Read the model definition and answer for the solid it produces. Units are mm, in the model's axes. A direction names the side the tool comes from. Coordinates: 2 decimals unless noted, no trailing zeros. Write each loop counter-clockwise with the first axis right and the second up, starting at its lowest first coordinate (ties: lowest second). Pieces come first, ordered by that corner, then holes. Notation, with made-up numbers: (62, 33.5) -> (113, 33.5) arc R22 ccw to (113, 64.5) -> close; hole circle Ø11 at (75.25, -11.75). An arc over 180 degrees is marked (long way). Return JSON: item names as keys, results as strings.
from build123d import *

# Parameters (mm, degrees)
SKETCH_1_W          = 28
SKETCH_1_H          = 31.376198505
SKETCH_1_R          = 1.25
EXTRUDE_1_DEPTH     = 4
SKETCH_4_R          = 2
EXTRUDE_3_DEPTH     = 3
SKETCH_6_R          = 2
EXTRUDE_4_DEPTH     = 24.38
SKETCH_7_W          = 28
SKETCH_7_H          = 2
CUT_EXTRUDE_1_DEPTH = 72


with BuildPart() as part:
    # 草图1 → 凸台-拉伸1 (new body)
    with BuildSketch(Plane.XY):
        with Locations((0, -1.688099253)):
            Rectangle(SKETCH_1_W, SKETCH_1_H)
        with Locations((-12, -12)):
            Circle(SKETCH_1_R, mode=Mode.SUBTRACT)
        with Locations((-12, 12)):
            Circle(SKETCH_1_R, mode=Mode.SUBTRACT)
        with Locations((12, 12)):
            Circle(SKETCH_1_R, mode=Mode.SUBTRACT)
        with Locations((12, -12)):
            Circle(SKETCH_1_R, mode=Mode.SUBTRACT)
    extrude(amount=EXTRUDE_1_DEPTH)

    # 草图4 → 凸台-拉伸3 (add)
    with BuildSketch(Plane(origin=(0, -17.376198505, 0), x_dir=(1, 0, 0), z_dir=(0, 1, 0))):
        with BuildLine():
            Line((-10.75, -4), (-16.6423045, -25.198978267))
            ThreePointArc((-16.6423045, -25.198978267), (-17.942800458, -27.122401454), (-20.139772651, -27.873507091))
            Line((-20.139772651, -27.873507091), (-24.991319672, -27.873507091))
            ThreePointArc((-24.991319672, -27.873507091), (-26.405533234, -27.287720654), (-26.991319672, -25.873507091))
            Line((-26.991319672, -25.873507091), (-26.991319672, -23.098090883))
            ThreePointArc((-26.991319672, -23.098090883), (-26.405533234, -21.68387732), (-24.991319672, -21.098090883))
            Line((-24.991319672, -21.098090883), (-20.272369191, -21.098090883))
            ThreePointArc((-20.272369191, -21.098090883), (-19.062245191, -20.690447597), (-18.345420115, -19.633690786))
            Line((-18.345420115, -19.633690786), (-14, -4))
            Line((-14, -4), (-10.75, -4))
        make_face()
        with Locations((-21, -24)):
            Circle(SKETCH_4_R, mode=Mode.SUBTRACT)
    extrude_3 = extrude(amount=EXTRUDE_3_DEPTH)

    # 草图6 → 凸台-拉伸4 (add)
    with BuildSketch(Plane(origin=(0, -14.376198505, 0), x_dir=(1, 0, 0), z_dir=(0, 1, 0))):
        with BuildLine():
            ThreePointArc((-20.272369191, -21.098090883), (-17.534000745, -22.331206649), (-16.6423045, -25.198978267))
            ThreePointArc((-16.6423045, -25.198978267), (-17.942800458, -27.122401454), (-20.139772651, -27.873507091))
            Line((-20.139772651, -27.873507091), (-24.991319672, -27.873507091))
            ThreePointArc((-24.991319672, -27.873507091), (-26.405533234, -27.287720654), (-26.991319672, -25.873507091))
            Line((-26.991319672, -25.873507091), (-26.991319672, -23.098090883))
            ThreePointArc((-26.991319672, -23.098090883), (-26.405533234, -21.68387732), (-24.991319672, -21.098090883))
            Line((-24.991319672, -21.098090883), (-20.272369191, -21.098090883))
        make_face()
        with Locations((-21, -24)):
            Circle(SKETCH_6_R, mode=Mode.SUBTRACT)
    extrude_4 = extrude(amount=EXTRUDE_4_DEPTH)

    # 镜向1: 凸台-拉伸3, 凸台-拉伸4 across plane
    add(extrude_3.mirror(Plane(origin=(0, 0, 0), x_dir=(0, 0, 1), z_dir=(1, 0, 0))))
    add(extrude_4.mirror(Plane(origin=(0, 0, 0), x_dir=(0, 0, 1), z_dir=(1, 0, 0))))

    # 草图7 → 切除-拉伸1 (cut)
    with BuildSketch(Plane(origin=(0, 14, 0), x_dir=(1, 0, 0), z_dir=(0, 1, 0))):
        with Locations((0, -1)):
            Rectangle(SKETCH_7_W, SKETCH_7_H)
    extrude(amount=-CUT_EXTRUDE_1_DEPTH, mode=Mode.SUBTRACT)


solid = part.part
1. Flat-ended cylindrical pins translate along their axes: pin 1 Ø3 at (x, y) = (12, -12) entering from +Z; pin 2 Ø12 at (y, z) = (10, 9.5) entering from -X; pin 3 Ø2 at (y, z) = (-8.5, 3.5) entering from +X; pin 4 Ø2 at (x, y) = (-12, 12) entering from +Z. Find the tip coordinate at first contact, or state that the pin passes through.
Taken from the geometry:
{"pin 1": "stops at z = 4", "pin 2": "stops at x = -14", "pin 3": "stops at x = 14", "pin 4": "passes through"}
2. For a pull along X with two mould halves and no side action, classify faces 3 (the face through (26.42, -3.88, 21.7)), 4 (the face through (11.84, 13.24, 2.99)), 5 (the face through (0, -1, 2)), 6 (the face through (-22.474, -3.878, 22.648)) as +X half, -X half, draft (parallel to the pull), parting line (faces both ways), or undercut.
Taken from the geometry:
{"face 3": "+X half", "face 4": "undercut", "face 5": "draft", "face 6": "undercut"}
3. A tool of negligible diameter and unlimited length cuts with its end or side. For faces 1 (the face through (-17.917, -3.878, 27.102)), 2 (the face through (-23, 10.004, 25)), from which of +Z, -Z, +X, -X, +Y, -Y can it reach the whole face along a straight path? Write none if from no direction.
Taken from the geometry:
{"face 1": "+Z, +Y, -Y", "face 2": "+Z, -Z, +X, -X, +Y"}
4. Consider L1, parallel to X at y = -12, z = 2.45; L2, parallel to Y at x = -12, z = 3.1; L3, parallel to Z at x = 21, y = -11. Determine where each line is inside the solid, lowest interval first.
Taken from the geometry:
{"L1": "x = -14 to -13.25, -10.75 to 10.75, 13.25 to 14", "L2": "y = -17.38 to -13.25, -10.75 to 10.75, 13.25 to 14", "L3": "z = 21.1 to 22, 26 to 27.87"}
5. The part is cut by section C-C (y = -12). Determine the outline of the cut face in (x, z), then the cut area to 3 significant figures.
Taken from the geometry:
{"outline": "(-26.99, 23.1) arc R2 ccw to (-24.99, 21.1) -> (-20.27, 21.1) arc R3.66 ccw to (-16.64, 25.2) arc R3.65 ccw to (-20.14, 27.87) -> (-24.99, 27.87) arc R2 ccw to (-26.99, 25.87) -> close; (-14, 2) -> (-13.25, 2) -> (-13.25, 4) -> (-14, 4) -> close; (-10.75, 2) -> (10.75, 2) -> (10.75, 4) -> (-10.75, 4) -> close; (13.25, 2) -> (14, 2) -> (14, 4) -> (13.25, 4) -> close; (16.64, 25.2) arc R3.66 ccw to (20.27, 21.1) -> (24.99, 21.1) arc R2 ccw to (26.99, 23.1) -> (26.99, 25.87) arc R2 ccw to (24.99, 27.87) -> (20.14, 27.87) arc R3.65 ccw to start; hole circle Ø4 at (-21, 24); hole circle Ø4 at (21, 24)", "area": "147 mm2"}
6. The part is cut by section A-A (y = 9). Determine the outline of the cut face in (x, z), then the cut area to 3 significant figures.
Taken from the geometry:
{"outline": "(-26.99, 23.1) arc R2 ccw to (-24.99, 21.1) -> (-20.27, 21.1) arc R3.66 ccw to (-16.64, 25.2) arc R3.65 ccw to (-20.14, 27.87) -> (-24.99, 27.87) arc R2 ccw to (-26.99, 25.87) -> close; (-14, 2) -> (14, 2) -> (14, 4) -> (-14, 4) -> close; (16.64, 25.2) arc R3.66 ccw to (20.27, 21.1) -> (24.99, 21.1) arc R2 ccw to (26.99, 23.1) -> (26.99, 25.87) arc R2 ccw to (24.99, 27.87) -> (20.14, 27.87) arc R3.65 ccw to start; hole circle Ø4 at (-21, 24); hole circle Ø4 at (21, 24)", "area": "157 mm2"}
7. The part is cut by section B-B (x = 21). Determine the outline of the cut face in (y, z), then the cut area to 3 significant figures.
Taken from the geometry:
{"outline": "(-17.38, 21.1) -> (10, 21.1) -> (10, 22) -> (-17.38, 22) -> close; (-17.38, 26) -> (10, 26) -> (10, 27.87) -> (-17.38, 27.87) -> close", "area": "76.0 mm2"}
8. The part is cut by section D-D (z = 18.25). Determine the outline of the cut face in (x, y).
Taken from the geometry:
{"outline": "(-17.96, -17.38) -> (-14.71, -17.38) -> (-14.71, -14.38) -> (-17.96, -14.38) -> close; (14.71, -17.38) -> (17.96, -17.38) -> (17.96, -14.38) -> (14.71, -14.38) -> close"}
